Could you check a few things on this drawing? It's one solid part, dimensions in mm from its lowest x, y, z. A direction names the side the tool comes from. Give positions to 0.01 mm unless a question says otherwise; leave off trailing zeros. Order: outer loops, then holes, each group sorted by start corner. A loop starts at its lowest first (then second) coordinate and runs counter-clockwise, first axis right, second up. Notation, with made-up numbers: (-30.75, 56) -> (-18.75, 56) arc R27 cw to (-18.75, 92) -> close; hole circle Ø5 at (-8.75, 70). An arc over 180 degrees is marked (long way). Answer as a JSON object with one key per item and string values.
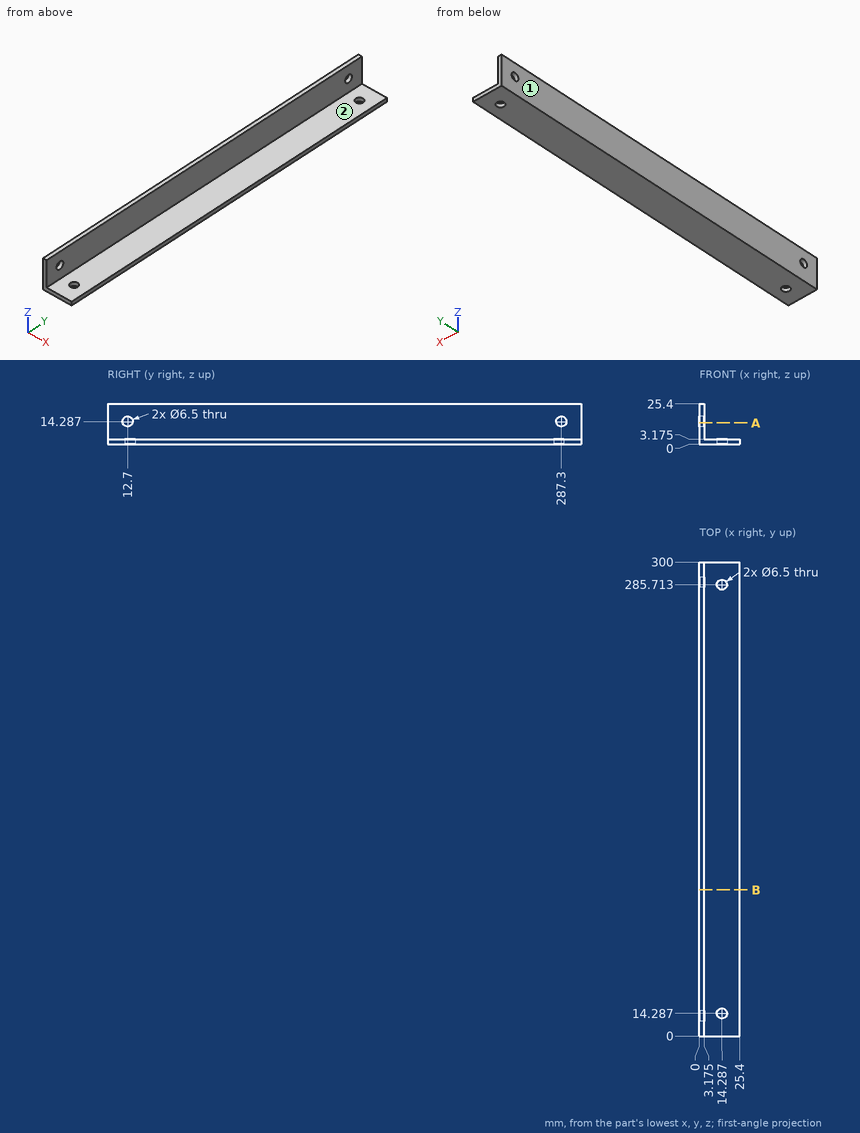
1. For the marked faces 1 and 2, which set-ups out of +Z, -Z, +X, -X, +Y, -Y let a thin tool reach every point of the face, with its end or its side?
Worked answers:
{"face 1": "+Z, -Z, -X, +Y, -Y", "face 2": "+Z, +X, +Y, -Y"}
2. Will these pins go through, and if not, where does the flat tip stop? pin 1 Ø5 at (y, z) = (12.7, 14.29) entering from -X; pin 2 Ø10 at (x, y) = (19.5, 266) entering from +Z (1 decimal); pin 3 Ø1 at (y, z) = (193, 21.5) entering from +X (1 decimal).
Worked answers:
{"pin 1": "through", "pin 2": "z = 3.2", "pin 3": "x = 3.2"}
3. Please list where these lines run through material, in increasing order: L1, parallel to Z at x = 1.2, y = 287.3; L2, parallel to X at y = 243.5, z = 18.5 (1 decimal).
Worked answers:
{"L1": "0 to 11.04, 17.54 to 25.4", "L2": "0 to 3.2"}
4. If we section it at B-B on y = 92.5: Please give me the cut outline in (x, z) (1 decimal), then the cut area to 3 significant figures.
Worked answers:
{"outline": "(0, 0) -> (25.4, 0) -> (25.4, 3.2) -> (3.2, 3.2) -> (3.2, 25.4) -> (0, 25.4) -> close", "area": "151 mm²"}
5. If we section it at A-A on z = 13.5: Please give me the cut outline in (x, y) (1 decimal).
Worked answers:
{"outline": "(0, 0) -> (3.2, 0) -> (3.2, 9.5) -> (0, 9.5) -> close; (0, 15.9) -> (3.2, 15.9) -> (3.2, 284.1) -> (0, 284.1) -> close; (0, 290.5) -> (3.2, 290.5) -> (3.2, 300) -> (0, 300) -> close"}
